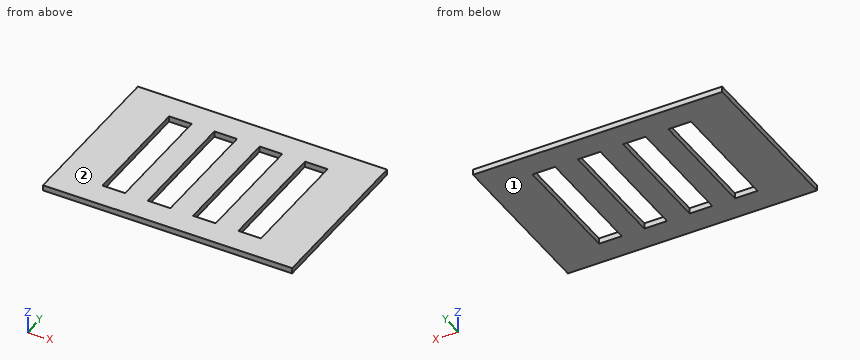
Autodesk Inventor part; units mm, degrees
ref_plane "YZ Plane" through (0, 0, 0) normal (1, 0, 0) x (0, 1, 0)
ref_plane "XZ Plane" through (0, 0, 0) normal (0, 1, 0) x (-1, 0, 0)
ref_plane "XY Plane" through (0, 0, 0) normal (0, 0, 1) x (1, 0, 0)
sketch "Sketch1" plane through (0, 0, 0) normal (0, 0, 1) x (1, 0, 0)
  line L0 (0, 0) -> (139.7, 0)
  line L1 (139.7, 0) -> (139.7, 127)
  line L2 (139.7, 127) -> (0, 127)
  line L3 (0, 127) -> (0, 0)
  dimension "d0" = 139.7
  dimension "d1" = 127
extrude "Extrusion1" add sketch "Sketch1" along normal blind 3.175
sketch "Sketch2" plane through (0, 0, 3.175) normal (0, 0, 1) x (1, 0, 0)
  line L0 (0, 0) -> (139.7, 0)
  line L1 (139.7, 0) -> (139.7, 127)
  line L2 (0, 0) -> (139.7, 0)
  line L3 (139.7, 0) -> (139.7, 19.05)
  line L4 (139.7, 19.05) -> (0, 19.05)
  line L5 (0, 19.05) -> (0, 0)
  line L6 (139.7, 127) -> (0, 127)
  line L7 (0, 127) -> (19.05, 127)
  line L8 (0, 86.1969) -> (0, 127)
  line L9 (0, 127) -> (139.7, 127)
  line L10 (139.7, 127) -> (139.7, 107.95)
  line L11 (139.7, 107.95) -> (0, 107.95)
  line L12 (0, 107.95) -> (0, 127)
  line L13 (0, 127) -> (19.05, 127)
  line L14 (19.05, 127) -> (19.05, 0)
  line L15 (19.05, 0) -> (0, 0)
  line L16 (0, 0) -> (0, 127)
  line L17 (139.7, 0) -> (120.65, 0)
  line L18 (120.65, 0) -> (120.65, 127)
  line L19 (120.65, 127) -> (139.7, 127)
  line L20 (139.7, 127) -> (139.7, 0)
  point P0 (19.05, 19.05)
  point P1 (19.05, 107.95)
  point P2 (120.65, 107.95)
  point P3 (120.65, 19.05)
  dimension "d4" = 19.05
  dimension "d6" = 19.05
  dimension "d7" = 19.05
extrude "Extrusion2" add sketch "Sketch2" along normal blind 3.175 contours L5 L4 L14 L0 | L14 L4 L18 L0 | L16 L8 L11 L14 L4 | L18 L4 L1 L0 | L18 L11 L1 L4 | L14 L6 L18 L11 | L11 L8 L6 L14 | L18 L6 L1 L11
sketch "Sketch3" plane through (0, 0, 0) normal (0, 0, -1) x (-1, 0, 0)
  line L0 (-19.05, 19.05) -> (-120.65, 19.05)
  line L1 (-120.65, 107.95) -> (-19.05, 107.95)
  line L2 (-25.4, 107.95) -> (-25.4, 19.05)
  line L3 (-19.05, 107.95) -> (-19.05, 19.05)
  line L4 (-38.1, 107.95) -> (-38.1, 19.05)
  line L5 (-114.3, 107.95) -> (-114.3, 19.05)
  line L6 (-101.6, 107.95) -> (-101.6, 19.05)
  line L7 (-120.65, 19.05) -> (-120.65, 107.95)
  line L8 (-88.9, 107.95) -> (-88.9, 19.05)
  line L9 (-50.8, 107.95) -> (-50.8, 19.05)
  line L10 (-76.2, 107.95) -> (-76.2, 19.05)
  line L11 (-63.5, 107.95) -> (-63.5, 19.05)
  line L12 (-130.7408, 107.95) -> (-4.1346, 107.95)
  line L13 (0, 127) -> (0, 0)
  line L14 (-128.9627, 19.05) -> (-12.6698, 19.05)
  line L15 (-128.9627, 30.48) -> (-12.6698, 30.48)
  line L16 (-130.7408, 96.52) -> (-4.1346, 96.52)
  point P0 (-25.4, 96.52)
  point P1 (-38.1, 96.52)
  point P2 (-38.1, 30.48)
  point P3 (-25.4, 30.48)
  point P4 (-50.8, 96.52)
  point P5 (-63.5, 96.52)
  point P6 (-63.5, 30.48)
  point P7 (-50.8, 30.48)
  point P8 (-76.2, 96.52)
  point P9 (-88.9, 96.52)
  point P10 (-88.9, 30.48)
  point P11 (-76.2, 30.48)
  point P12 (-101.6, 96.52)
  point P13 (-114.3, 96.52)
  point P14 (-114.3, 30.48)
  point P15 (-101.6, 30.48)
  dimension "d14" = 12.7
  dimension "d15" = 6.35
  dimension "d17" = 12.7
  dimension "d18" = 12.7
  dimension "d19" = 12.7
  dimension "d20" = 12.7
  dimension "d21" = 12.7
  dimension "d22" = 12.7
  dimension "d23" = 11.43
  dimension "d24" = 11.43
extrude "Extrusion3" cut sketch "Sketch3" against normal through all contours L15 L4 L16 L2 | L15 L11 L16 L9 | L15 L8 L16 L10 | L15 L5 L16 L6
sketch "Sketch4" plane through (0, 0, 0) normal (0, 0, -1) x (-1, 0, 0)
  line L0 (-120.65, 19.05) -> (-120.65, 107.95)
  line L1 (-120.65, 107.95) -> (-19.05, 107.95)
  line L2 (-19.05, 107.95) -> (-19.05, 19.05)
  line L3 (-19.05, 19.05) -> (-120.65, 19.05)
  line L4 (-139.7, 127) -> (0, 127)
  line L5 (0, 0) -> (-139.7, 0)
  line L6 (-157.0502, 127) -> (65.2705, 127)
  line L7 (-157.0502, 110.49) -> (65.2705, 110.49)
  line L8 (-152.5949, 0) -> (41.6573, 0)
  line L9 (-152.5949, 16.51) -> (41.6573, 16.51)
  line L10 (-147.9168, 24.0704) -> (-145.2436, -7.3397)
  line L11 (8.7478, 21.5847) -> (14.9253, -14.4682)
  line L12 (-146.5802, 130.3299) -> (-146.5802, 103.3752)
  line L13 (-146.5802, 103.3752) -> (-146.5802, 100.0337)
  line L14 (14.9253, 133.2259) -> (10.47, 95.1328)
  point P0 (12.4462, 0)
  point P1 (9.6173, 16.51)
  point P2 (-147.2734, 16.51)
  point P3 (-145.8683, 0)
  point P4 (12.2662, 110.49)
  point P5 (14.1972, 127)
  point P6 (0, 127)
  point P7 (-146.5802, 127)
  point P8 (-146.5802, 110.49)
  dimension "d27" = 127
  dimension "d28" = 16.51
  dimension "d29" = 16.51
extrude "Extrusion4" cut sketch "Sketch4" against normal through all contours L4 L6 L14 L7 L12 | L5 L8 L10 L9 L11
sketch "Sketch6" plane through (139.7, 16.51, 0) normal (1, 0, 0) x (0, 0, -1)
  line L0 (-6.35, 0) -> (-6.35, 93.98)
  line L1 (-6.35, 93.98) -> (-3.175, 93.98)
  line L2 (-3.175, 93.98) -> (-3.175, -1176.02)
  line L3 (-3.175, -1176.02) -> (-6.35, -1176.02)
  line L4 (-6.35, -1176.02) -> (-6.35, 93.98)
  point P0 (0, -16.51)
  dimension "d32" = 3.175
  dimension "d33" = 1270
extrude "Extrusion5" cut sketch "Sketch6" against normal through all
sketch "Sketch7" plane through (0, 0, 3.175) normal (0, 0, 1) x (1, 0, 0)
  point P0 (0, 0)
sketch "Sketch8" plane through (0, 0, 3.175) normal (0, 0, 1) x (1, 0, 0)
  line L0 (114.3, 96.52) -> (114.3, 30.48)
  line L1 (139.7, 110.49) -> (139.7, 16.51)
  point P0 (0, 0)
  dimension "d36" = 25.4
properties part number "frount plate"
Geometry: final body of the model. Coordinates: model frame, mm. Face numbers are marked on the shaded views. Round coordinates to 2 decimals unless told otherwise and drop trailing zeros. Write each loop counter-clockwise with the first axis right and the second up, starting at its lowest first coordinate (ties: lowest second). Pieces come first, ordered by that corner, then holes.
Item 1: Mould query, pull axis Z, two halves, no side actions, for the marked faces 1 and 2. Classes: +Z half, -Z half, draft (parallel to the pull), parting line (faces both ways), or undercut.
Item 2: Section query A-A (x = 59.5). Return loops of the section in (y, z) (3 decimals).
Item 3: Material intervals for L1, parallel to X at y = 76, z = 0.95; L2, parallel to Y at x = 31, z = 1.4, sorted ascending.
Item 4: Section query B-B (y = 41). Return loops of the section in (x, z) (3 decimals), plus the area to 3 significant figures.
Item 5: Section query C-C (z = 1.45). Return loops of the section in (x, y), plus the area to 3 significant figures.
Completed:
1. face 1: -Z half
1. face 2: +Z half
2. outline: (16.51, 0) - (30.48, 0) - (30.48, 3.175) - (16.51, 3.175) - close; (96.52, 0) - (110.49, 0) - (110.49, 3.175) - (96.52, 3.175) - close
3. L1: x = 0 to 25.4, 38.1 to 50.8, 63.5 to 76.2, 88.9 to 101.6, 114.3 to 139.7
3. L2: y = 16.51 to 30.48, 96.52 to 110.49
4. outline: (0, 0) - (25.4, 0) - (25.4, 3.175) - (0, 3.175) - close; (38.1, 0) - (50.8, 0) - (50.8, 3.175) - (38.1, 3.175) - close; (63.5, 0) - (76.2, 0) - (76.2, 3.175) - (63.5, 3.175) - close; (88.9, 0) - (101.6, 0) - (101.6, 3.175) - (88.9, 3.175) - close; (114.3, 0) - (139.7, 0) - (139.7, 3.175) - (114.3, 3.175) - close
4. area: 282 mm2
5. outline: (0, 16.51) - (139.7, 16.51) - (139.7, 110.49) - (0, 110.49) - close; hole (25.4, 30.48) - (38.1, 30.48) - (38.1, 96.52) - (25.4, 96.52) - close; hole (50.8, 30.48) - (63.5, 30.48) - (63.5, 96.52) - (50.8, 96.52) - close; hole (76.2, 30.48) - (88.9, 30.48) - (88.9, 96.52) - (76.2, 96.52) - close; hole (101.6, 30.48) - (114.3, 30.48) - (114.3, 96.52) - (101.6, 96.52) - close
5. area: 9,770 mm2
